from build123d import *

# Parameters (mm, degrees)
F0_W     = 127.0000040531
F0_H     = 97.6745411754
F0_R     = 24.3083232654
F0_R_2   = 17.1484022814
F1_DEPTH = 25.4
F2_DEPTH = 50.8
F3_DEPTH = 76.2


with BuildPart() as f1:
    # F0 (on Top) → F1 (new body)
    with BuildSketch(Plane.XY):
        Rectangle(F0_W, F0_H)
        Circle(F0_R, mode=Mode.SUBTRACT)
        Circle(F0_R)
        Circle(F0_R_2, mode=Mode.SUBTRACT)
    extrude(amount=F1_DEPTH)

    # F0 (on Top) → F2 (join)
    with BuildSketch(Plane.XY):
        Rectangle(F0_W, F0_H)
        Circle(F0_R, mode=Mode.SUBTRACT)
    extrude(amount=F2_DEPTH)

    # F3 (add): a face of the model
    f3_faces = [f1.faces().sort_by_distance(p)[0] for p in [
        (-23.6207800566, 0, 25.4),
    ]]
    extrude(f3_faces, amount=F3_DEPTH)


solid = f1.part
Design review of the part built by this model. Coordinates are the model's own, in mm. A direction names the side the tool comes from. Round coordinates to 2 decimals unless told otherwise and drop trailing zeros. Loops run counter-clockwise (first coordinate to the right, second up) from the corner with the lowest first, then second, coordinate; pieces in that order, holes last. Notation, with made-up numbers: (-22.5, 30.25) -> (24.5, 30.25) arc R20 ccw to (24.5, 61.25) -> close; hole circle Ø7 at (-27, 75). An arc over 180 degrees is marked (long way). Use one line per item in the form item = value. Start each with the question number.
Q1. We need section B-B on x = 0. Give the boundary of the cut face in (y, z), then the cut area to 3 significant figures.
Q2. Wall thickness on line 1 along Z through (x, y) = (-1, 42); line 2 along Y through (x, z) = (-15, 10.5); line 3 along X through (y, z) = (13, 24): over which ranges is each line inside the solid? List them lowest first. Write a range as [from, to].
Q3. We need section C-C on z = 25.5. Give the boundary of the cut face in (x, y), then the cut area to 3 significant figures.
Q4. We need section A-A on y = 0. Give the boundary of the cut face in (x, z).
Q5. For pin 1 Ø8 at (x, z) = (22, 62) entering from +Y; pin 2 Ø2 at (x, z) = (-41, 52.5) entering from -Y; pin 3 Ø10 at (x, y) = (-48, -3) entering from -Z, all flat-tipped, find the tip position at first contact; note any pin that passes through.
Q6. Draft analysis for pull direction X (two halves, no side actions). For faces 3 (the face through (-15, 22, 50.8)), 4 (the face through (16.357, 5.151, 50.089)), 5 (the face through (63.5, -1, 25)), state which applies: +X half, -X half, draft (parallel to the pull), parting line (faces both ways), or undercut.
Q7. Machinability: for faces 1 (the face through (5, 17, 101.6)), 2 (the face through (-19.29, 14.79, 75.84)), which of the approach directions +Z, -Z, +X, -X, +Y, -Y give a long, thin tool a straight path to every point of the face, cutting with its end or side? Answer none if there is none.
Q8. We need section D-D on x = 31. Give the boundary of the cut face in (y, z), then the cut area to 3 significant figures.
Calculated:
q1.outline = (-48.84, 0) -> (-17.15, 0) -> (-17.15, 101.6) -> (-24.31, 101.6) -> (-24.31, 50.8) -> (-48.84, 50.8) -> close; (17.15, 0) -> (48.84, 0) -> (48.84, 50.8) -> (24.31, 50.8) -> (24.31, 101.6) -> (17.15, 101.6) -> close
q1.area = 3,950 mm²
q2.line_1 = [0, 50.8]
q2.line_2 = [-48.84, -8.31], [8.31, 48.84]
q2.line_3 = [-63.5, -11.18], [11.18, 63.5]
q3.outline = (-63.5, -48.84) -> (63.5, -48.84) -> (63.5, 48.84) -> (-63.5, 48.84) -> close; hole circle Ø34.3 at (0, 0)
q3.area = 11,500 mm²
q4.outline = (-63.5, 0) -> (-17.15, 0) -> (-17.15, 101.6) -> (-24.31, 101.6) -> (-24.31, 50.8) -> (-63.5, 50.8) -> close; (17.15, 0) -> (63.5, 0) -> (63.5, 50.8) -> (24.31, 50.8) -> (24.31, 101.6) -> (17.15, 101.6) -> close
q5.pin_1 = 16.34
q5.pin_2 = through
q5.pin_3 = 0
q6.face_3 = draft
q6.face_4 = undercut
q6.face_5 = +X half
q7.face_1 = +Z, +X, -X, +Y, -Y
q7.face_2 = +Z
q8.outline = (-48.84, 0) -> (48.84, 0) -> (48.84, 50.8) -> (-48.84, 50.8) -> close
q8.area = 4,960 mm²
